CAD build for the part. Positions are in the model's coordinates, mm. A direction names the side the tool comes from. Coordinates: 2 decimals unless noted, no trailing zeros. Write each loop counter-clockwise with the first axis right and the second up, starting at its lowest first coordinate (ties: lowest second). Pieces come first, ordered by that corner, then holes. Notation, with made-up numbers: (42, 45) - (89, 45) arc R12 cw to (89, 54) - close; hole circle Ø7 at (-17.5, -36). An arc over 180 degrees is marked (long way). Answer in a Markdown table with one row per item. Add a question column.
Q1. Band-saw the part on B-B (z = 6.75). List the corners of the cut face in (x, y), and give its area (3 significant figures).
Q2. Drill centre lines: line 1 along Y through (x, z) = (14, 5); line 2 along Y through (x, z) = (-2, 4); line 3 along X through (y, z) = (9, 3.25). Where is each one in solid material? Low to high. Write a range as from..to.
Q3. Band-saw the part on D-D (x = -33). List the corners of the cut face in (y, z).
Q4. Band-saw the part on C-C (y = 9). List the corners of the cut face in (x, z).
Q5. Two-plate mould, pull along Y, no slides. Class faces 1 (the flat face through (-1, -22, 0)), 2 (the cylindrical face through (47.69, 15.02, 7.4)), 3 (the flat face through (17.248, -10.126, 7.395)), 4 (the flat face through (0, -20, 7)): +Y half, -Y half, draft (parallel to the pull), parting line (faces both ways), or undercut.
Q6. Band-saw the part on A-A (x = 0). List the corners of the cut face in (y, z), and give its area (3 significant figures).
Q7. Pin check, flat tips, straight feed: pin 1 (6 mm diameter, centred on x = -18.5, z = 6.5, fed in from +Y); pin 2 (1.5 mm diameter, centred on y = 34.5, z = 11, fed in from +X); pin 3 (7.5 mm diameter, centred on x = 1, z = 8, fed in from -Y); pin 4 (2 mm diameter, centred on x = 37, y = 23.5, fed in from -Z). Stop position of each tip, or through.
Q8. 3-axis set-ups, long thin cutter, end or side, ignore diameter. For faces 5 (the flat face through (-1, -22, 15)), 6 (the flat face through (-17.393, -9.874, 7.395)): which of +Z, -Z, +X, -X, +Y, -Y reach the whole face in a straight line?
```python
from build123d import *

# Parameters (mm, degrees)
SKETCH1_R           = 50
BOSS_EXTRUDE2_DEPTH = 15
FILLET1_R           = 2


with BuildPart() as part:
    # Sketch1 → Boss-Extrude2 (new body)
    with BuildSketch(Plane.XY):
        Circle(SKETCH1_R)
        Polygon((23.094010768, 0), (11.547005384, 20), (-11.547005384, 20), (-23.094010768, 0), (-11.547005384, -20), (11.547005384, -20), align=None, mode=Mode.SUBTRACT)
    extrude(amount=BOSS_EXTRUDE2_DEPTH)

    # Fillet1
    fillet1_edges = [part.edges().sort_by_distance(p)[0] for p in [
        (23.094010768, 0, 7.5),
        (11.547005384, 20, 7.5),
        (-11.547005384, 20, 7.5),
        (-23.094010768, 0, 7.5),
        (-11.547005384, -20, 7.5),
        (11.547005384, -20, 7.5),
    ]]
    fillet(fillet1_edges, radius=FILLET1_R)


solid = part.part
```
Checked values:
| question | item | result |
|---|---|---|
| 1 | outline | circle Ø100 at (0, 0); hole (-22.52, -1) - (-12.12, -19) arc R2 ccw to (-10.39, -20) - (10.39, -20) arc R2 ccw to (12.12, -19) - (22.52, -1) arc R2 ccw to (22.52, 1) - (12.12, 19) arc R2 ccw to (10.39, 20) - (-10.39, 20) arc R2 ccw to (-12.12, 19) - (-22.52, 1) arc R2 ccw to start |
| 1 | area | 6,470 mm² |
| 2 | line 1 | y = -48..-15.75, 15.75..48 |
| 2 | line 2 | y = -49.96..-20, 20..49.96 |
| 2 | line 3 | x = -49.18..-17.9, 17.9..49.18 |
| 3 | outline | (-37.56, 0) - (37.56, 0) - (37.56, 15) - (-37.56, 15) - close |
| 4 | outline | (-49.18, 0) - (-17.9, 0) - (-17.9, 15) - (-49.18, 15) - close; (17.9, 0) - (49.18, 0) - (49.18, 15) - (17.9, 15) - close |
| 5 | face 1 | draft |
| 5 | face 2 | parting line |
| 5 | face 3 | undercut |
| 5 | face 4 | undercut |
| 6 | outline | (-50, 0) - (-20, 0) - (-20, 15) - (-50, 15) - close; (20, 0) - (50, 0) - (50, 15) - (20, 15) - close |
| 6 | area | 900 mm² |
| 7 | pin 1 | stops at y = 47.54 |
| 7 | pin 2 | stops at x = 36.89 |
| 7 | pin 3 | stops at y = -50 |
| 7 | pin 4 | stops at z = 0 |
| 8 | face 5 | +Z, +X, -X, +Y, -Y |
| 8 | face 6 | +Z, -Z |
